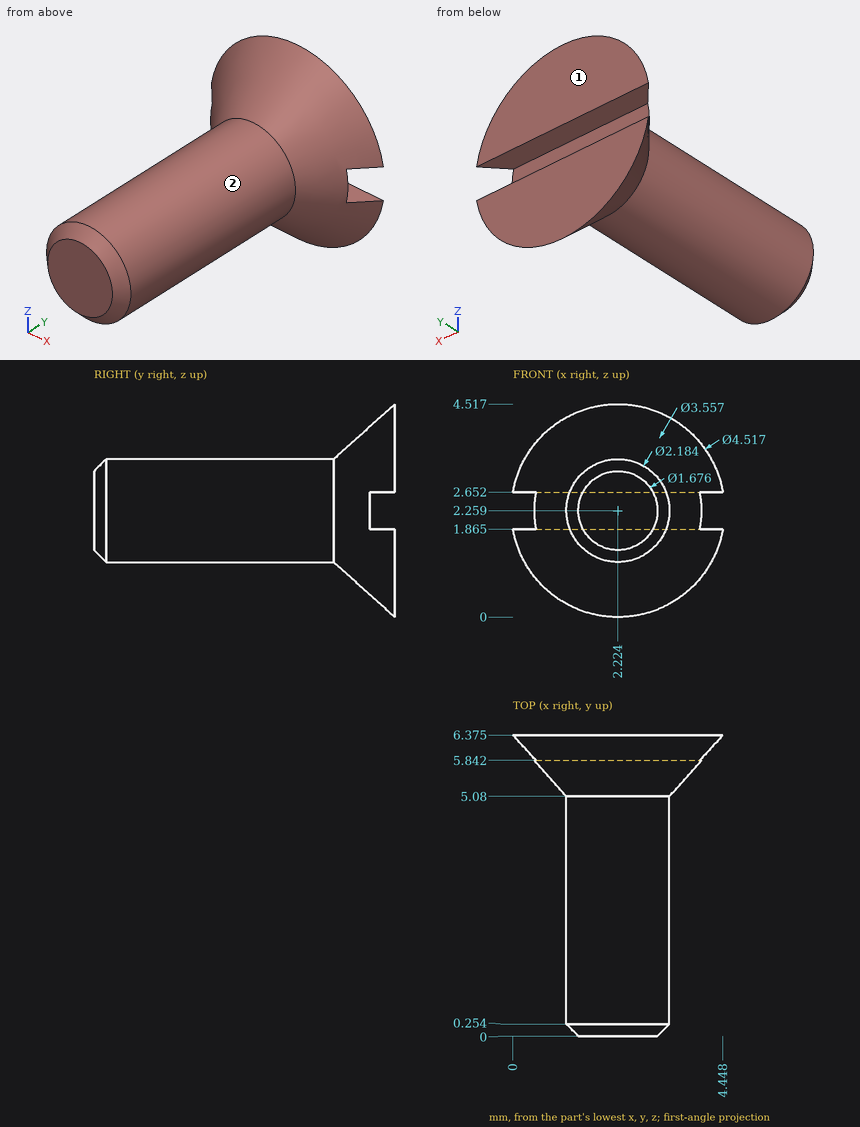
Could you check a few things on this drawing? It's one solid part, dimensions in mm from its lowest x, y, z. Coordinates: 2 decimals unless noted, no trailing zeros. Answer as a JSON object with one key per item and string values. Group by question number.
Q1. Will these pins go through, and if not, where does the flat tip stop? P1, Ø0.6, axis at x = 3, y = 6, coming from the -Z side; P2, Ø1.5, axis at x = 2, z = 0.5, coming from the -Y side (1 decimal).
Q2. I need wall thicknesses on line 1 (X direction, y = 4, z = 2.3) (1 decimal); line 2 (Z direction, x = 3.05, y = 3.25) (1 decimal); line 3 (Y direction, x = 1.3, z = 0.75) (1 decimal). Which ranges of each line are inside material? Lowest first, please. Write a range as from..to.
Q3. We'd pull the mould along Z, two halves only. Please class the marked faces 1 and 2: +Z half, -Z half, draft (parallel to the pull), parting line (faces both ways), or undercut.
Determined:
{
 "1": {"P1": "stops at z = 0.19", "P2": "stops at y = 0.2"},
 "2": {"line 1": "x = 1.1..3.3", "line 2": "z = 1.5..3", "line 3": "y = 5.8..6.4"},
 "3": {"face 1": "draft", "face 2": "parting line"}
}
